```python
from build123d import *

# Parameters (mm, degrees)
SKETCH_W     = 105
SKETCH_H     = 75
PAD_DEPTH    = 2.5
PAD001_DEPTH = 10
SKETCH002_R  = 1.5
POCKET_DEPTH = 5.001


with BuildPart() as part:
    # Sketch → Pad (new body)
    with BuildSketch(Plane.XY):
        with Locations((52.5, 37.5)):
            Rectangle(SKETCH_W, SKETCH_H)
    extrude(amount=PAD_DEPTH)

    # Sketch001 → Pad001 (new body)
    with BuildSketch(Plane.XY.offset(2.5)):
        Polygon((5, 0), (5, 5), (23, 5), (23, 65), (83, 65), (83, 55), (33, 55), (33, 5), (55, 5), (55, 0), align=None)
    extrude(amount=PAD001_DEPTH)

    # Sketch002 → Pocket (cut, through all)
    with BuildSketch(Plane(origin=(0, 5, 0), x_dir=(-1, 0, 0), z_dir=(0, 1, 0))):
        with Locations((-12.5, 7.5)):
            Circle(SKETCH002_R)
        with Locations((-47.5, 7.5)):
            Circle(SKETCH002_R)
    extrude(amount=-POCKET_DEPTH, mode=Mode.SUBTRACT)


solid = part.part
```
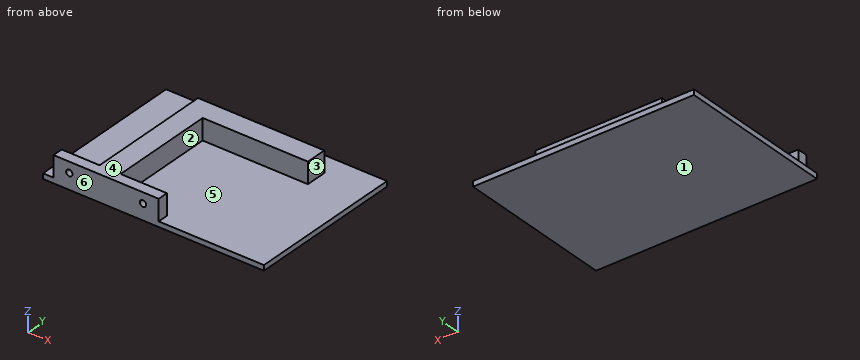
Model file for the job. Use its own axes, mm. Face numbers are marked on the shaded views. A direction names the side the tool comes from. Give positions to 0.01 mm unless a question says otherwise; leave off trailing zeros. Loops run counter-clockwise (first coordinate to the right, second up) from the corner with the lowest first, then second, coordinate; pieces in that order, holes last. Notation, with made-up numbers: (3, 87) - (18, 87) arc R33 cw to (18, 122) - close; hole circle Ø11 at (1.5, -35.75). An arc over 180 degrees is marked (long way). One line per item, written item: value. Start each with the question number.
1. Which spindle directions (+Z, -Z, +X, -X, +Y, -Y) get a long thin tool onto all of the face, cutting with end or side? Do the marked faces 1, 2 and 3. Say none if no direction does.
2. Pull direction Y, two halves, no side cores. Call the marked faces 4, 5 and 6: pulls with the +Y half, pulls with the -Y half, needs draft (parallel to the pull), parting line crosses it, or undercut.
3. Slice it at A-A (x = 47.5). List the corners of the cut face in (y, z).
4. Slice it at B-B (z = 7.5). List the corners of the cut face in (x, y), plus the area to 3 significant figures.
5. Slice it at C-C (y = 58). List the corners of the cut face in (x, z).
6. Slice it at D-D (x = 24.5). List the corners of the cut face in (y, z).
7. Probe L1, parallel to Y at x = 45.5, z = 3.25; L2, parallel to Z at x = 47.5, y = 4.5; L3, parallel to Z at x = 61.5, y = 8. List the from-to ranges inside material, lowest first. Write a range as from..to.
8. Pin check, flat tips, straight feed: pin 1 (5 mm diameter, centred on x = 60, z = 8.5, fed in from +Y); pin 2 (6 mm diameter, centred on x = 31, z = 8, fed in from -Y); pin 3 (1 mm diameter, centred on y = 25.5, z = 7, fed in from +X); pin 4 (2.5 mm diameter, centred on y = 3, z = 9, fed in from -X). Stop position of each tip, or through.
Solution:
1. face 1: -Z, +X, -X, +Y, -Y
1. face 2: +Z, +X
1. face 3: +Z, +X, +Y, -Y
2. face 4: needs draft
2. face 5: undercut
2. face 6: pulls with the -Y half
3. outline: (0, 0) - (75, 0) - (75, 2.5) - (65, 2.5) - (65, 12.5) - (55, 12.5) - (55, 2.5) - (5, 2.5) - (5, 6) - (0, 6) - close; (0, 9) - (5, 9) - (5, 12.5) - (0, 12.5) - close
4. outline: (5, 0) - (11, 0) - (11, 5) - (5, 5) - close; (14, 0) - (46, 0) - (46, 5) - (33, 5) - (33, 55) - (83, 55) - (83, 65) - (23, 65) - (23, 5) - (14, 5) - close; (49, 0) - (55, 0) - (55, 5) - (49, 5) - close
4. area: 1,320 mm^2
5. outline: (0, 0) - (105, 0) - (105, 2.5) - (83, 2.5) - (83, 12.5) - (23, 12.5) - (23, 2.5) - (0, 2.5) - close
6. outline: (0, 0) - (75, 0) - (75, 2.5) - (65, 2.5) - (65, 12.5) - (0, 12.5) - close
7. L1: y = 0..5, 55..65
7. L2: z = 0..6, 9..12.5
7. L3: z = 0..2.5
8. pin 1: stops at y = 65
8. pin 2: stops at y = 0
8. pin 3: stops at x = 33
8. pin 4: stops at x = 5
